Geometry: final body of the model. Coordinates: model frame, mm. Round coordinates to 2 decimals unless told otherwise and drop trailing zeros. Write each loop counter-clockwise with the first axis right and the second up, starting at its lowest first coordinate (ties: lowest second). Pieces come first, ordered by that corner, then holes.
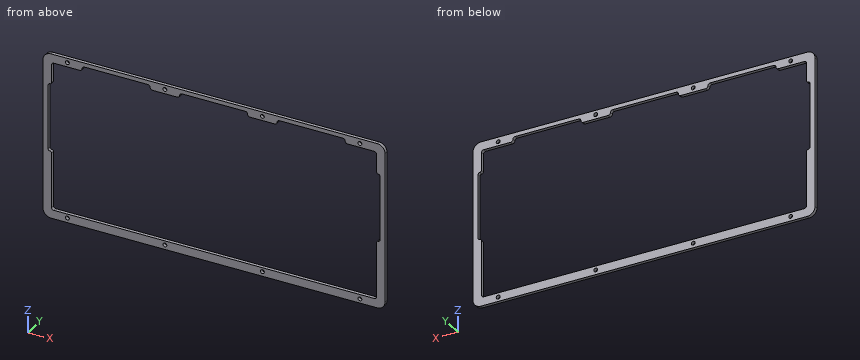
from build123d import *

# Parameters (mm, degrees)
SKETCH1_W           = 350
SKETCH1_H           = 200
BOSS_EXTRUDE1_DEPTH = 3
SKETCH2_W           = 350
SKETCH2_H           = 200
SKETCH2_R           = 1.7
CUT_EXTRUDE2_DEPTH  = 3


with BuildPart() as part:
    # Sketch1 → Boss-Extrude1 (new body)
    with BuildSketch(Plane(origin=(0, 0, 0), x_dir=(1, 0, 0), z_dir=(0, 1, 0))):
        with Locations((175, 100)):
            Rectangle(SKETCH1_W, SKETCH1_H)
    extrude(amount=BOSS_EXTRUDE1_DEPTH)

    # Sketch2 → Cut-Extrude2 (cut)
    with BuildSketch(Plane(origin=(0, 3, 0), x_dir=(1, 0, 0), z_dir=(0, 1, 0))):
        with Locations((175, 100)):
            Rectangle(SKETCH2_W, SKETCH2_H)
        with BuildLine():
            ThreePointArc((18.78172506, 5.694207131), (13.831977592, 7.744459663), (11.78172506, 12.694207131))
            Line((11.78172506, 12.694207131), (11.78172506, 142.893667131))
            ThreePointArc((11.78172506, 142.893667131), (13.831977592, 147.843414599), (18.78172506, 149.893667131))
            Line((18.78172506, 149.893667131), (306.48107506, 149.893667131))
            ThreePointArc((306.48107506, 149.893667131), (311.430822528, 147.843414599), (313.48107506, 142.893667131))
            Line((313.48107506, 142.893667131), (313.48107506, 12.694207131))
            ThreePointArc((313.48107506, 12.694207131), (311.430822528, 7.744459663), (306.48107506, 5.694207131))
            Line((306.48107506, 5.694207131), (18.78172506, 5.694207131))
        make_face(mode=Mode.SUBTRACT)
        with Locations(Location((119.28172506, 145.893667131, 0), (0, 0, 270))):
            Circle(SKETCH2_R)
        with Locations(Location((33.28172506, 145.893667131, 0), (0, 0, 270))):
            Circle(SKETCH2_R)
        with Locations(Location((205.28172506, 145.893667131, 0), (0, 0, 270))):
            Circle(SKETCH2_R)
        with Locations(Location((291.28172506, 146.143667131, 0), (0, 0, 270))):
            Circle(SKETCH2_R)
        with Locations(Location((119.28172506, 9.444207131, 0), (0, 0, 270))):
            Circle(SKETCH2_R)
        with Locations(Location((33.28172506, 9.444207131, 0), (0, 0, 270))):
            Circle(SKETCH2_R)
        with Locations(Location((205.28172506, 9.444207131, 0), (0, 0, 270))):
            Circle(SKETCH2_R)
        with Locations(Location((291.28172506, 9.694207131, 0), (0, 0, 270))):
            Circle(SKETCH2_R)
        with BuildLine():
            ThreePointArc((46.28172506, 11.194207131), (46.867511498, 9.779993569), (48.28172506, 9.194207131))
            Line((48.28172506, 9.194207131), (104.28172506, 9.194207131))
            ThreePointArc((104.28172506, 9.194207131), (105.695938623, 9.779993569), (106.28172506, 11.194207131))
            ThreePointArc((106.28172506, 11.194207131), (106.867511498, 12.608420694), (108.28172506, 13.194207131))
            Line((108.28172506, 13.194207131), (130.28172506, 13.194207131))
            ThreePointArc((130.28172506, 13.194207131), (131.695938623, 12.608420694), (132.28172506, 11.194207131))
            ThreePointArc((132.28172506, 11.194207131), (132.867511498, 9.779993569), (134.28172506, 9.194207131))
            Line((134.28172506, 9.194207131), (190.28172506, 9.194207131))
            ThreePointArc((190.28172506, 9.194207131), (191.695938623, 9.779993569), (192.28172506, 11.194207131))
            ThreePointArc((192.28172506, 11.194207131), (192.867511498, 12.608420694), (194.28172506, 13.194207131))
            Line((194.28172506, 13.194207131), (216.28172506, 13.194207131))
            ThreePointArc((216.28172506, 13.194207131), (217.695938623, 12.608420694), (218.28172506, 11.194207131))
            ThreePointArc((218.28172506, 11.194207131), (218.867511498, 9.779993569), (220.28172506, 9.194207131))
            Line((220.28172506, 9.194207131), (276.28172506, 9.194207131))
            ThreePointArc((276.28172506, 9.194207131), (277.695938623, 9.779993569), (278.28172506, 11.194207131))
            ThreePointArc((278.28172506, 11.194207131), (278.867511498, 12.608420694), (280.28172506, 13.194207131))
            Line((280.28172506, 13.194207131), (303.98107506, 13.194207131))
            ThreePointArc((303.98107506, 13.194207131), (305.395288623, 13.779993569), (305.98107506, 15.194207131))
            Line((305.98107506, 15.194207131), (305.98107506, 30.694207131))
            ThreePointArc((305.98107506, 30.694207131), (306.420414888, 31.754867303), (307.48107506, 32.194207131))
            ThreePointArc((307.48107506, 32.194207131), (308.541735232, 32.633546959), (308.98107506, 33.694207131))
            Line((308.98107506, 33.694207131), (308.98107506, 89.694207131))
            ThreePointArc((308.98107506, 89.694207131), (308.541735232, 90.754867303), (307.48107506, 91.194207131))
            ThreePointArc((307.48107506, 91.194207131), (306.420414888, 91.633546959), (305.98107506, 92.694207131))
            Line((305.98107506, 92.694207131), (305.98107506, 140.393667131))
            ThreePointArc((305.98107506, 140.393667131), (305.395288623, 141.807880694), (303.98107506, 142.393667131))
            Line((303.98107506, 142.393667131), (21.28172506, 142.393667131))
            ThreePointArc((21.28172506, 142.393667131), (19.867511498, 141.807880694), (19.28172506, 140.393667131))
            Line((19.28172506, 140.393667131), (19.28172506, 92.694207131))
            ThreePointArc((19.28172506, 92.694207131), (18.842385232, 91.633546959), (17.78172506, 91.194207131))
            ThreePointArc((17.78172506, 91.194207131), (16.721064888, 90.754867303), (16.28172506, 89.694207131))
            Line((16.28172506, 89.694207131), (16.28172506, 33.694207131))
            ThreePointArc((16.28172506, 33.694207131), (16.721064888, 32.633546959), (17.78172506, 32.194207131))
            ThreePointArc((17.78172506, 32.194207131), (18.842385232, 31.754867303), (19.28172506, 30.694207131))
            Line((19.28172506, 30.694207131), (19.28172506, 15.194207131))
            ThreePointArc((19.28172506, 15.194207131), (19.867511498, 13.779993569), (21.28172506, 13.194207131))
            Line((21.28172506, 13.194207131), (44.28172506, 13.194207131))
            ThreePointArc((44.28172506, 13.194207131), (45.695938623, 12.608420694), (46.28172506, 11.194207131))
        make_face()
    extrude(amount=-CUT_EXTRUDE2_DEPTH, mode=Mode.SUBTRACT)


solid = part.part
1) Line query: probe 1 along Z at (x, y) = (137, 2); probe 2 along X at (y, z) = (0.4, -64); probe 3 along X at (y, z) = (1.2, -132). Output: solid intervals per line, ascending.
2) Section A-A on z = -101. Output: boundary loops of the cut face in (x, y).
3) Section C-C on y = 0.55. State how many separate pieces and enclosed holes the cut face has, plus the area to 3 significant figures.
4) Section B-B on x = 175. Output: boundary loops of the cut face in (y, z).
Filled in:
1. probe 1: z = -149.89 to -142.39, -9.19 to -5.69
1. probe 2: x = 11.78 to 16.28, 308.98 to 313.48
1. probe 3: x = 11.78 to 19.28, 305.98 to 313.48
2. outline: (11.78, 0) - (19.28, 0) - (19.28, 3) - (11.78, 3) - close; (305.98, 0) - (313.48, 0) - (313.48, 3) - (305.98, 3) - close
3. separate pieces: 1
3. enclosed holes: 9
3. area: 5,280 mm2
4. outline: (0, -149.89) - (3, -149.89) - (3, -142.39) - (0, -142.39) - close; (0, -9.19) - (3, -9.19) - (3, -5.69) - (0, -5.69) - close
